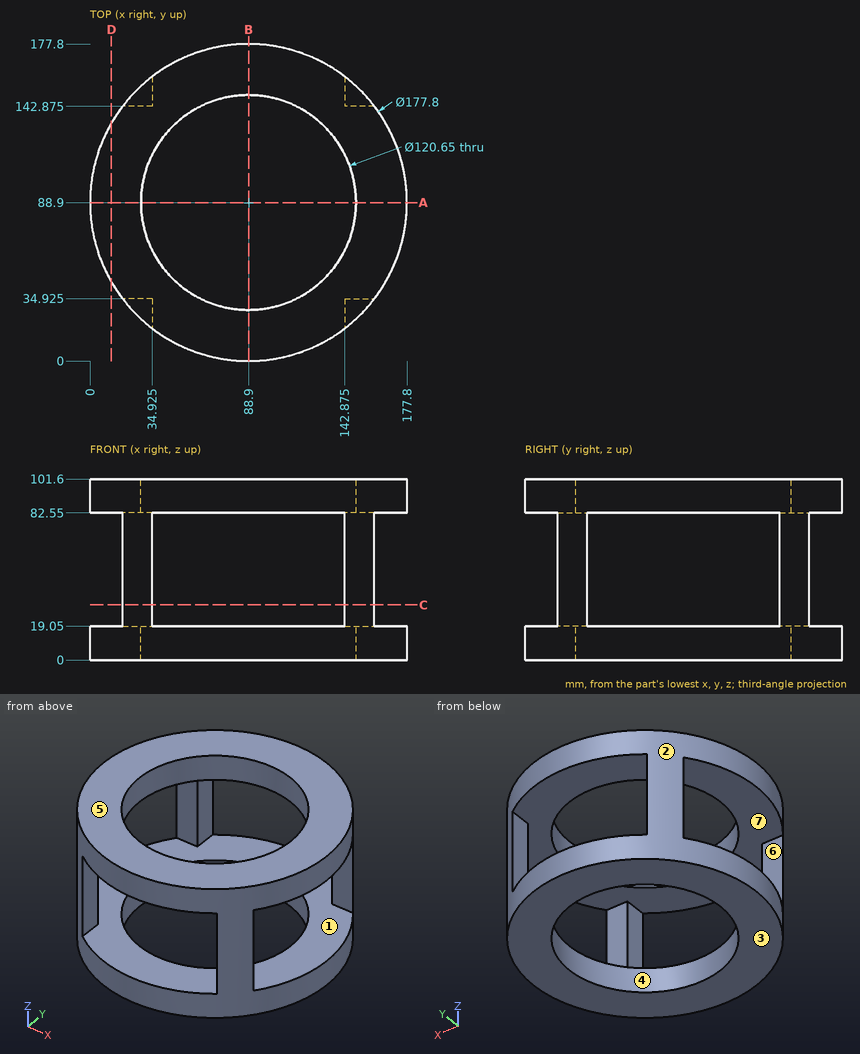
Here's the drawing with two shaded views (mm, measured from the low corner). I have some questions. A direction names the side the tool comes from. Round coordinates to 2 decimals unless told otherwise and drop trailing zeros. Loops run counter-clockwise (first coordinate to the right, second up) from the corner with the lowest first, then second, coordinate; pieces in that order, holes last. Notation, with made-up numbers: M 48,42.25 L 69,42.25 A11 ccw 69,49.25 Z; hole C 31.25,49 d7. An arc over 180 degrees is marked long. Answer as CSV lines item,"result".
1) Imagine slicing it at D-D on x = 12. List the corners of the cut face in (y, z) for me.
From the geometry:
outline,"M 44.3,0 L 133.5,0 L 133.5,19.05 L 44.3,19.05 Z; M 44.3,82.55 L 133.5,82.55 L 133.5,101.6 L 44.3,101.6 Z"
2) Imagine slicing it at A-A on y = 88.9. List the corners of the cut face in (x, z) for me (3 decimals).
From the geometry:
outline,"M 0,0 L 28.575,0 L 28.575,19.05 L 0,19.05 Z; M 0,82.55 L 28.575,82.55 L 28.575,101.6 L 0,101.6 Z; M 149.225,0 L 177.8,0 L 177.8,19.05 L 149.225,19.05 Z; M 149.225,82.55 L 177.8,82.55 L 177.8,101.6 L 149.225,101.6 Z"
3) Which directions (+Z, -Z, +X, -X, +Y, -Y) give clear straight access to the entire face, cutting with the end or side of a thin tool? Please do the marked faces 5, 6 and 7.
From the geometry:
face 5,"+Z, +X, -X, +Y, -Y"
face 6,"+X, -X"
face 7,"none"
4) For pin 1 Ø8.5 at (x, z) = (29, 49) entering from +Y; pin 2 Ø5 at (x, z) = (152.5, 36) entering from +Y; pin 3 Ø13.5 at (x, z) = (26, 65.5) entering from -Y; pin 4 Ø4 at (x, z) = (48.5, 80) entering from -Y, each with a flat end and sliding along its axis, tell me the tip position at first contact or that it passes through.
From the geometry:
pin 1,"y = 158.23"
pin 2,"y = 153.48"
pin 3,"y = 19.98"
pin 4,"through"
5) We'd pull the mould along X, two halves only. Please class the marked faces 1, 2, 3 and 4: released by +X, released by -X, zero draft, split by the parting line, or undercut.
From the geometry:
face 1,"undercut"
face 2,"split by the parting line"
face 3,"zero draft"
face 4,"undercut"
6) If I drill on probe 1 along Y at (x, z) = (88, 5); probe 2 along Z at (x, y) = (22, 73.5); probe 3 along X at (y, z) = (129.5, 86), over which ranges is the centre line in solid material (lowest first)?
From the geometry:
probe 1,"0 to 28.58, 149.22 to 177.8"
probe 2,"0 to 19.05, 82.55 to 101.6"
probe 3,"9.81 to 44.28, 133.52 to 167.99"
7) Imagine slicing it at C-C on z = 31. List the corners of the cut face in (x, y) for me (3 decimals), and give its area (3 significant figures).
From the geometry:
outline,"M 18.261,34.925 A88.9 ccw 34.925,18.261 L 34.925,34.925 Z; M 18.261,142.875 L 34.925,142.875 L 34.925,159.539 A88.9 ccw Z; M 142.875,18.261 A88.9 ccw 159.539,34.925 L 142.875,34.925 Z; M 142.875,142.875 L 159.539,142.875 A88.9 ccw 142.875,159.539 Z"
area,"605 mm^2"
